```python
from build123d import *

# Parameters (mm, degrees)
SKETCH1_R           = 10.922
BOSS_EXTRUDE1_DEPTH = 127
SKETCH2_R           = 10.414
CUT_EXTRUDE1_DEPTH  = 124.46
CUT_EXTRUDE2_DEPTH  = 15.24
SKETCH5_R           = 2.590245468
BOSS_EXTRUDE2_DEPTH = 12.7


with BuildPart() as part:
    # Sketch1 → Boss-Extrude1 (new body)
    with BuildSketch(Plane.XY):
        Circle(SKETCH1_R)
    extrude(amount=BOSS_EXTRUDE1_DEPTH)

    # Sketch2 → Cut-Extrude1 (cut)
    with BuildSketch(Plane.XY.offset(127)):
        Circle(SKETCH2_R)
    extrude(amount=-CUT_EXTRUDE1_DEPTH, mode=Mode.SUBTRACT)

    # Sketch4 → Cut-Extrude2 (cut)
    with BuildSketch(Plane(origin=(0, 0, 0), x_dir=(0, 0, -1), z_dir=(1, 0, 0))):
        with BuildLine():
            Line((-114.3, 5.067588244), (-12.7, 5.067588244))
            ThreePointArc((-12.7, 5.067588244), (-7.632411756, 0), (-12.7, -5.067588244))
            Line((-12.7, -5.067588244), (-114.3, -5.067588244))
            ThreePointArc((-114.3, -5.067588244), (-119.367588244, 0), (-114.3, 5.067588244))
        make_face()
    extrude(amount=CUT_EXTRUDE2_DEPTH, mode=Mode.SUBTRACT)

    # Sketch5 → Boss-Extrude2 (add)
    with BuildSketch(Plane(origin=(0, 0, 0), x_dir=(0, 0, -1), z_dir=(1, 0, 0))):
        with Locations((-3.984592514, 0)):
            Circle(SKETCH5_R)
    extrude(amount=BOSS_EXTRUDE2_DEPTH)


solid = part.part
```
Input: part model. Units: mm. Frame: model coordinates. A direction names the side the tool comes from. Give positions to 0.01 mm unless a question says otherwise; leave off trailing zeros. Loops run counter-clockwise (first coordinate to the right, second up) from the corner with the lowest first, then second, coordinate; pieces in that order, holes last.
1) Section query D-D on y = 7. Return the cut outline in (x, z), and give its area (3 significant figures).
A:
outline: (-8.38, 0) - (8.38, 0) - (8.38, 127) - (7.71, 127) - (7.71, 2.54) - (-7.71, 2.54) - (-7.71, 127) - (-8.38, 127) - close
area: 210 mm2
2) Section query B-B on x = 6.5. Return the cut outline in (y, z).
A:
outline: (-8.78, 0) - (8.78, 0) - (8.78, 127) - (8.14, 127) - (8.14, 2.54) - (2.15, 2.54) arc R2.59 ccw (long way) to (-2.15, 2.54) - (-8.14, 2.54) - (-8.14, 127) - (-8.78, 127) - close
3) Mould query, pull axis X, two halves, no side actions, for faces 3 (the cylindrical face through (5.134, 0.078, 6.574)), 4 (the flat face through (12.7, 0, 4)), 5 (the cylindrical face through (-10.91, 0.48, 62.61)), 6 (the flat face through (0, 0, 5)). Classes: released by +X, released by -X, zero draft, split by the parting line, or undercut.
A:
face 3: undercut
face 4: released by +X
face 5: split by the parting line
face 6: undercut
4) Line query: L1, parallel to Y at x = 0, z = 49.5; L2, parallel to Z at x = -6.25, y = -3.75; L3, parallel to X at y = 7.25, z = 31.5. Output: solid intervals per line, ascending.
A:
L1: y = -10.92 to -10.41, 10.41 to 10.92
L2: z = 0 to 2.54
L3: x = -8.17 to -7.48, 7.48 to 8.17
5) Contact query for flat-ended pins moving along their axis: pin 1 (12 mm diameter, centred on y = 8, z = 49.5, fed in from -X); pin 2 (8 mm diameter, centred on y = 8.5, z = 41, fed in from -X); pin 3 (6 mm diameter, centred on x = 1, y = -4, fed in from +Z). Output: stop coordinate, or through.
A:
pin 1: stops at x = -10.74
pin 2: stops at x = -9.95
pin 3: stops at z = 6.37
6) Section query C-C on z = 28.5. Return the cut outline in (x, y), and give its area (3 significant figures).
A:
outline: (9.1, -5.07) arc R10.41 cw (long way) to (9.1, 5.07) - (9.68, 5.07) arc R10.92 ccw (long way) to (9.68, -5.07) - close
area: 28.7 mm2
7) Reachability of faces 1 (the flat face through (10, -4, 127)), 2 (the cylindrical face through (10.681, 0.037, 7.633)) from +Z, -Z, +X, -X, +Y, -Y: full face, straight path, thin tool, end or side. Return the list, or none.
A:
face 1: +Z, +X, -X, +Y, -Y
face 2: +X
8) Section query A-A on y = -8. Return the cut outline in (x, z).
A:
outline: (-7.44, 0) - (7.44, 0) - (7.44, 127) - (6.67, 127) - (6.67, 2.54) - (-6.67, 2.54) - (-6.67, 127) - (-7.44, 127) - close
